from build123d import *

# Parameters (mm, degrees)
SKETCH1_R             = 1
BOSS_EXTRUDE1_DEPTH   = 2
BOSS_EXTRUDE2_DEPTH   = 23
BOSS_EXTRUDE2_2_DEPTH = 23
BOSS_EXTRUDE3_DEPTH   = 2
FILLET1_R             = 2.5
FILLET2_R             = 1.5


with BuildPart() as part:
    # Sketch1 → Boss-Extrude1 (new body)
    with BuildSketch(Plane.XY):
        with BuildLine():
            Line((-1.914568893, 0), (-53.034632217, 0))
            ThreePointArc((-53.034632217, 0), (-54.430407674, 0.574584772), (-55.017150852, 1.965292948))
            Line((-55.017150852, 1.965292948), (-55.500249363, 57.322899279))
            ThreePointArc((-55.500249363, 57.322899279), (-55.399437354, 57.964587872), (-55.09663904, 58.539253421))
            Line((-55.09663904, 58.539253421), (-45.118252169, 71.678754712))
            ThreePointArc((-45.118252169, 71.678754712), (-44.186512298, 72.353695471), (-43.03683386, 72.39755554))
            Line((-43.03683386, 72.39755554), (0.580818713, 60.968995882))
            ThreePointArc((0.580818713, 60.968995882), (1.66875601, 60.234846813), (2.059695099, 58.981950551))
            Line((2.059695099, 58.981950551), (0.066817491, 1.913402589))
            ThreePointArc((0.066817491, 1.913402589), (-0.537343288, 0.556435263), (-1.914568893, 0))
        make_face()
        with Locations((-27.474600555, 5)):
            Circle(SKETCH1_R, mode=Mode.SUBTRACT)
        with Locations((-22.474600555, 11.5)):
            Circle(SKETCH1_R, mode=Mode.SUBTRACT)
        with Locations((-32.474600555, 11.5)):
            Circle(SKETCH1_R, mode=Mode.SUBTRACT)
        with Locations((-6.292158567, 6.135518638)):
            Circle(SKETCH1_R, mode=Mode.SUBTRACT)
        with Locations((-50.206815558, 6.135518638)):
            Circle(SKETCH1_R, mode=Mode.SUBTRACT)
        with Locations((-50.206815558, 56.218481747)):
            Circle(SKETCH1_R, mode=Mode.SUBTRACT)
        with Locations((-4.635001699, 53.732746446)):
            Circle(SKETCH1_R, mode=Mode.SUBTRACT)
    extrude(amount=BOSS_EXTRUDE1_DEPTH)



with BuildPart() as body_2:
    # Sketch2 → Boss-Extrude2 (new body)
    with BuildSketch(Plane(origin=(0, 0, 0), x_dir=(-1, 0, 0), z_dir=(0, 0, -1))):
        Polygon((-4.001759752, 32.322899279), (-1.128740515, 32.322899279), (-2.001759752, 57.322899279), (-4.001759752, 57.322899279), align=None)
    extrude(amount=BOSS_EXTRUDE2_DEPTH)


with BuildPart() as body_3:
    # Sketch2 → Boss-Extrude2 2 (new body)
    with BuildSketch(Plane(origin=(0, 0, 0), x_dir=(-1, 0, 0), z_dir=(0, 0, -1))):
        Polygon((57.500249363, 57.322899279), (55.500249363, 57.322899279), (55.282077669, 32.322899279), (57.500249363, 32.322899279), align=None)
    extrude(amount=BOSS_EXTRUDE2_2_DEPTH)


with BuildPart() as part_1:
    add(part.part)

    add(body_2.part)  # Boss-Extrude3 merges body 2

    add(body_3.part)  # Boss-Extrude3 merges body 3
    # Sketch3 → Boss-Extrude3 (add)
    with BuildSketch(Plane.XY):
        Polygon((-57.500249363, 57.322899279), (-55.500249363, 57.322899279), (-55.282077669, 32.322899279), (-57.500249363, 32.322899279), align=None)
        Polygon((2.001759752, 57.322899279), (4.001759752, 57.322899279), (4.001759752, 32.322899279), (1.128740515, 32.322899279), align=None)
    extrude(amount=BOSS_EXTRUDE3_DEPTH)

    # Fillet1
    fillet1_edges = [part_1.edges().sort_by_distance(p)[0] for p in [
        (4.001759752, 44.822899279, 2),
        (-57.500249363, 44.822899279, 2),
    ]]
    fillet(fillet1_edges, radius=FILLET1_R)

    # Fillet2
    fillet2_edges = [part_1.edges().sort_by_distance(p)[0] for p in [
        (3.001759752, 57.322899279, -23),
        (2.565250134, 32.322899279, -23),
        (-56.500249363, 57.322899279, -23),
        (-56.391163516, 32.322899279, -23),
    ]]
    fillet(fillet2_edges, radius=FILLET2_R)


solid = part_1.part
Could you check a few things on this model? Use its own coordinates, in mm. Round coordinates to 2 decimals unless told otherwise and drop trailing zeros. Order: outer loops, then holes, each group sorted by start corner. A loop starts at its lowest first (then second) coordinate and runs counter-clockwise, first axis right, second up.
(1) Imagine slicing it at B-B (y = 11.5). Write out the boundary of the cut face in (x, z), plus the area to 3 significant figures.
Response values:
outline: (-55.1, 0) - (-33.47, 0) - (-33.47, 2) - (-55, 2) arc R2.5 ccw to (-55.1, 2) - close; (-31.47, 0) - (-23.47, 0) - (-23.47, 2) - (-31.47, 2) - close; (-21.47, 0) - (0.4, 0) - (0.4, 2) - (-21.47, 2) - close
area: 103 mm2
(2) I'm going to push flat-ended pins straight in: pin 1 (2.5 mm diameter, centred on x = -4.64, y = 53.73, fed in from -Z); pin 2 (1.8 mm diameter, centred on x = -22.47, y = 11.5, fed in from +Z); pin 3 (1.6 mm diameter, centred on x = 3, z = -13, fed in from +Y); pin 4 (2.5 mm diameter, centred on x = -56, z = -11, fed in from -Y). Where does each tip first touch, or does it pass through?
Response values:
pin 1: stops at z = 0
pin 2: passes through
pin 3: stops at y = 57.32
pin 4: stops at y = 32.32
(3) Imagine slicing it at D-D (x = -18). Write out the boundary of the cut face in (y, z), plus the area to 3 significant figures.
Response values:
outline: (0, 0) - (65.84, 0) - (65.84, 2) - (0, 2) - close
area: 132 mm2
(4) If we mould it in two halves opening along Y, with no side actions, what happens to faces 1 (the cylindrical face through (-44.2, 72.35, 0.99)), 2 (the cylindrical face through (-49.253, 6.436, 0.986)), 3 (the flat face through (-57.5, 45, -12))? For each: released by +Y, released by -Y, zero draft, split by the parting line, or undercut.
Response values:
face 1: released by +Y
face 2: undercut
face 3: zero draft
(5) Imagine slicing it at A-A (z = -16.5). Write out the boundary of the cut face in (x, y).
Response values:
outline: (-57.5, 32.32) - (-55.28, 32.32) - (-55.5, 57.32) - (-57.5, 57.32) - close; (1.13, 32.32) - (4, 32.32) - (4, 57.32) - (2, 57.32) - close
(6) Please list where these lines run through material, in increasing order: line 1 along Z through (x, y) = (-3, 3); line 2 along X through (y, z) = (35, -1); line 3 along Y through (x, z) = (-45, 0.5).
Response values:
line 1: z = 0 to 2
line 2: x = -57.5 to -55.31, 1.22 to 4
line 3: y = 0 to 71.82
(7) Imagine slicing it at C-C (y = 42.5). Write out the boundary of the cut face in (x, z), plus the area to 3 significant figures.
Response values:
outline: (-57.5, -23) - (-55.37, -23) - (-55.37, 0) - (1.48, 0) - (1.48, -23) - (4, -23) - (4, -0.5) arc R2.5 ccw to (1.5, 2) - (-55, 2) arc R2.5 ccw to (-57.5, -0.5) - close
area: 227 mm2
